from build123d import *

# Parameters (mm, degrees)
BOSS_EXTRUDE1_DEPTH                             = 20
SKETCH2_R                                       = 3
CUT_EXTRUDE1_DEPTH                              = 48.244047244
SKETCH3_R                                       = 3
CUT_EXTRUDE2_DEPTH                              = 55.120236511
SKETCH4_W                                       = 4
SKETCH4_H                                       = 3
CUT_EXTRUDE3_DEPTH                              = 43.201895692
CUT_EXTRUDE4_REACH                              = 56.12
SKETCH5_R                                       = 1.5
CUT_EXTRUDE5_REACH                              = 56.12
SKETCH6_R                                       = 1.5
CUT_EXTRUDE6_REACH                              = 51.558
SKETCH7_R                                       = 1.5
CSK_FOR_M3_FLAT_HEAD_MACHINE_SCREW1_D           = 3.4
CSK_FOR_M3_FLAT_HEAD_MACHINE_SCREW1_DEPTH       = 4
CSK_FOR_M3_FLAT_HEAD_MACHINE_SCREW1_CSINK_D     = 6.3
CSK_FOR_M3_FLAT_HEAD_MACHINE_SCREW1_CSINK_ANGLE = 90
SKETCH9_R                                       = 0.75
CUT_EXTRUDE7_DEPTH                              = 50.558046773


with BuildPart() as part:
    # Sketch1 → Boss-Extrude1 (new body)
    with BuildSketch(Plane(origin=(0, 0, 0), x_dir=(0, 0, -1), z_dir=(1, 0, 0))):
        Polygon((-15, 0), (-15, 14), (15, 14), (15, 0), (11, 0), (11, 10), (-11, 10), (-11, 0), (-11, -30), (11, -30), (11, -20), (15, -20), (15, -34), (-15, -34), (-15, -20), align=None)
    extrude(amount=BOSS_EXTRUDE1_DEPTH)

    # Sketch2 → Cut-Extrude1 (cut, through all)
    with BuildSketch(Plane(origin=(0, 0, 11), x_dir=(-1, 0, 0), z_dir=(0, 0, -1))):
        with Locations(Location((-10, -10, 0), (0, 0, 90))):
            Circle(SKETCH2_R)
    extrude(amount=-CUT_EXTRUDE1_DEPTH, mode=Mode.SUBTRACT)

    # Sketch3 → Cut-Extrude2 (cut, through all)
    with BuildSketch(Plane(origin=(0, 14, 0), x_dir=(1, 0, 0), z_dir=(0, 1, 0))):
        with Locations(Location((10, 0, 0), (0, 0, 270))):
            Circle(SKETCH3_R)
    extrude(amount=-CUT_EXTRUDE2_DEPTH, mode=Mode.SUBTRACT)

    # Sketch4 → Cut-Extrude3 (cut, through all)
    with BuildSketch(Plane(origin=(20, 0, 0), x_dir=(0, 0, -1), z_dir=(1, 0, 0))):
        with Locations((13, 1.5)):
            Rectangle(SKETCH4_W, SKETCH4_H)
        with Locations((13, -21.5)):
            Rectangle(SKETCH4_W, SKETCH4_H)
    extrude(amount=-CUT_EXTRUDE3_DEPTH, mode=Mode.SUBTRACT)

    # Sketch5 → Cut-Extrude4 (cut, up to next)
    with BuildSketch(Plane.XZ.offset(34), mode=Mode.PRIVATE) as cut_extrude4_sk1:
        with Locations(Location((9.864597697, 6.998690322, 0), (0, 0, 270))):
            Circle(SKETCH5_R)
    cut_extrude4_tool1 = extrude(cut_extrude4_sk1.sketch, amount=-CUT_EXTRUDE4_REACH, mode=Mode.PRIVATE) & part.part
    # Sketch5 → Cut-Extrude4 (cut, up to next)
    with BuildSketch(Plane.XZ.offset(34), mode=Mode.PRIVATE) as cut_extrude4_sk2:
        with Locations(Location((10.135402303, -6.998690322, 0), (0, 0, 270))):
            Circle(SKETCH5_R)
    cut_extrude4_tool2 = extrude(cut_extrude4_sk2.sketch, amount=-CUT_EXTRUDE4_REACH, mode=Mode.PRIVATE) & part.part
    add(cut_extrude4_tool1.solids().sort_by_distance((9.864598, -34, 6.99869))[0], mode=Mode.SUBTRACT)
    add(cut_extrude4_tool2.solids().sort_by_distance((10.135402, -34, -6.99869))[0], mode=Mode.SUBTRACT)

    # Sketch6 → Cut-Extrude5 (cut, up to next)
    with BuildSketch(Plane(origin=(0, 14, 0), x_dir=(1, 0, 0), z_dir=(0, 1, 0)), mode=Mode.PRIVATE) as cut_extrude5_sk1:
        with Locations(Location((17.679589652, 4.193614525, 0), (0, 0, 270))):
            Circle(SKETCH6_R)
    cut_extrude5_tool1 = extrude(cut_extrude5_sk1.sketch, amount=-CUT_EXTRUDE5_REACH, mode=Mode.PRIVATE) & part.part
    # Sketch6 → Cut-Extrude5 (cut, up to next)
    with BuildSketch(Plane(origin=(0, 14, 0), x_dir=(1, 0, 0), z_dir=(0, 1, 0)), mode=Mode.PRIVATE) as cut_extrude5_sk2:
        with Locations(Location((2.320410348, -4.193614525, 0), (0, 0, 270))):
            Circle(SKETCH6_R)
    cut_extrude5_tool2 = extrude(cut_extrude5_sk2.sketch, amount=-CUT_EXTRUDE5_REACH, mode=Mode.PRIVATE) & part.part
    add(cut_extrude5_tool1.solids().sort_by_distance((17.67959, 14, -4.193615))[0], mode=Mode.SUBTRACT)
    add(cut_extrude5_tool2.solids().sort_by_distance((2.32041, 14, 4.193615))[0], mode=Mode.SUBTRACT)

    # Sketch7 → Cut-Extrude6 (cut, up to next)
    with BuildSketch(Plane(origin=(0, 0, -15), x_dir=(-1, 0, 0), z_dir=(0, 0, -1)), mode=Mode.PRIVATE) as cut_extrude6_sk1:
        with Locations((-15, 6.5)):
            Circle(SKETCH7_R)
    cut_extrude6_tool1 = extrude(cut_extrude6_sk1.sketch, amount=-CUT_EXTRUDE6_REACH, mode=Mode.PRIVATE) & part.part
    # Sketch7 → Cut-Extrude6 (cut, up to next)
    with BuildSketch(Plane(origin=(0, 0, -15), x_dir=(-1, 0, 0), z_dir=(0, 0, -1)), mode=Mode.PRIVATE) as cut_extrude6_sk2:
        with Locations((-5, 6.5)):
            Circle(SKETCH7_R)
    cut_extrude6_tool2 = extrude(cut_extrude6_sk2.sketch, amount=-CUT_EXTRUDE6_REACH, mode=Mode.PRIVATE) & part.part
    cut_extrude6_1 = cut_extrude6_tool1.solids().sort_by_distance((15, 6.5, -15))[0]
    add(cut_extrude6_1, mode=Mode.SUBTRACT)
    cut_extrude6_2 = cut_extrude6_tool2.solids().sort_by_distance((5, 6.5, -15))[0]
    add(cut_extrude6_2, mode=Mode.SUBTRACT)
    cut_extrude6 = cut_extrude6_1 + cut_extrude6_2  # Cut-Extrude6 as one shape, for the pattern or mirror that repeats it

    # CSK for M3 Flat Head Machine Screw1
    with Locations(Plane(origin=(5, 6.5, -11), x_dir=(0, 1, 0), z_dir=(0, 0, 1))):
        with Locations((0, 0), (0, -10)):
            csk_for_m3_flat_head_machine_screw1 = CounterSinkHole(CSK_FOR_M3_FLAT_HEAD_MACHINE_SCREW1_D / 2, CSK_FOR_M3_FLAT_HEAD_MACHINE_SCREW1_CSINK_D / 2, depth=CSK_FOR_M3_FLAT_HEAD_MACHINE_SCREW1_DEPTH, counter_sink_angle=CSK_FOR_M3_FLAT_HEAD_MACHINE_SCREW1_CSINK_ANGLE)

    # Mirror1: Cut-Extrude6, CSK for M3 Flat Head Machine Screw1 across plane
    add(cut_extrude6.mirror(Plane.ZX.offset(-10)), mode=Mode.SUBTRACT)
    add(csk_for_m3_flat_head_machine_screw1.mirror(Plane.ZX.offset(-10)), mode=Mode.SUBTRACT)

    # Sketch9 → Cut-Extrude7 (cut, through all)
    with BuildSketch(Plane.XY.offset(15)):
        with Locations((5.5, -10)):
            Circle(SKETCH9_R)
        with Locations((14.5, -10)):
            Circle(SKETCH9_R)
    extrude(amount=-CUT_EXTRUDE7_DEPTH, mode=Mode.SUBTRACT)


solid = part.part
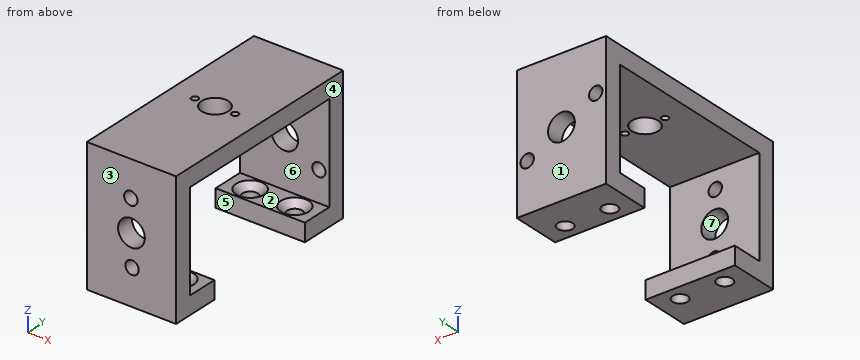
Geometry check sheet. Reference: the model listing, model coordinates, mm. Face numbers are marked on the shaded views. A direction names the side the tool comes from. Coordinates: 2 decimals unless noted, no trailing zeros. Order: outer loops, then holes, each group sorted by start corner. A loop starts at its lowest first (then second) coordinate and runs counter-clockwise, first axis right, second up. Notation, with made-up numbers: (12, -14) -> (28, -14) arc R23 cw to (28, -6) -> close; hole circle Ø8 at (39, 45). An arc over 180 degrees is marked (long way). Use a Markdown table: item, result. Add a question column.
1. Set-up check for the marked faces 5, 6 and 7: record each of +Z, -Z, +X, -X, +Y, -Y from which the full face is reachable in a straight line by a thin tool's end or side.
2. Material ranges on L1, parallel to X at y = 6.5, z = -13.1; L2, parallel to Y at x = 12.75, z = -3.75; L3, parallel to X at y = 12.95, z = 0, recorded low to high.
3. Cross-section at C-C (z = -5). Enter the section's corners in (x, y).
4. Mould release check, pull along Y, two halves, no side actions. Record for the marked faces 1, 2, 3 and 4: pulls with the +Y half, pulls with the -Y half, needs draft (parallel to the pull), parting line crosses it, or undercut.
5. Cross-section at D-D (y = 6.5). Enter the section's corners in (x, z).
6. Go/stop test with flat-tipped pins: pin 1 Ø3 at (x, y) = (7, -7.5) entering from -Z; pin 2 Ø5.5 at (x, y) = (10, -10) entering from -Z. Record where each tip stops, or that it passes through.
7. Cross-section at B-B (z = 0). Enter the section's corners in (x, y), and give its area (3 significant figures).
8. Cross-section at A-A (y = -10). Enter the section's corners in (x, z).
Filled sheet:
| question | item | result |
|---|---|---|
| 1 | face 5 | -Z, +X, -X |
| 1 | face 6 | +X, -X |
| 1 | face 7 | +Y, -Y |
| 2 | L1 | 0 to 3.3, 6.7 to 13.3, 16.7 to 20 |
| 2 | L2 | -34 to -30, 10 to 14 |
| 2 | L3 | 0 to 7, 13 to 20 |
| 3 | outline | (0, -34) -> (20, -34) -> (20, -30) -> (0, -30) -> close; (0, 10) -> (16.41, 10) -> (16.41, 14) -> (0, 14) -> close; (18.94, 10) -> (20, 10) -> (20, 14) -> (18.94, 14) -> close |
| 4 | face 1 | pulls with the +Y half |
| 4 | face 2 | undercut |
| 4 | face 3 | pulls with the -Y half |
| 4 | face 4 | needs draft |
| 5 | outline | (0, -15) -> (3.3, -15) -> (3.3, -12.45) -> (1.85, -11) -> (0, -11) -> close; (0, 11) -> (20, 11) -> (20, 15) -> (0, 15) -> close; (6.7, -15) -> (13.3, -15) -> (13.3, -12.45) -> (11.85, -11) -> (8.15, -11) -> (6.7, -12.45) -> close; (16.7, -15) -> (20, -15) -> (20, -11) -> (18.15, -11) -> (16.7, -12.45) -> close |
| 6 | pin 1 | z = 11 |
| 6 | pin 2 | through |
| 7 | outline | (0, -34) -> (7, -34) -> (7, -30) -> (0, -30) -> close; (0, 10) -> (7, 10) -> (7, 14) -> (0, 14) -> close; (13, -34) -> (20, -34) -> (20, -30) -> (13, -30) -> close; (13, 10) -> (20, 10) -> (20, 14) -> (13, 14) -> close |
| 7 | area | 112 mm2 |
| 8 | outline | (0, 11) -> (4.75, 11) -> (4.75, 15) -> (0, 15) -> close; (6.25, 11) -> (7, 11) -> (7, 15) -> (6.25, 15) -> close; (13, 11) -> (13.75, 11) -> (13.75, 15) -> (13, 15) -> close; (15.25, 11) -> (20, 11) -> (20, 15) -> (15.25, 15) -> close |
